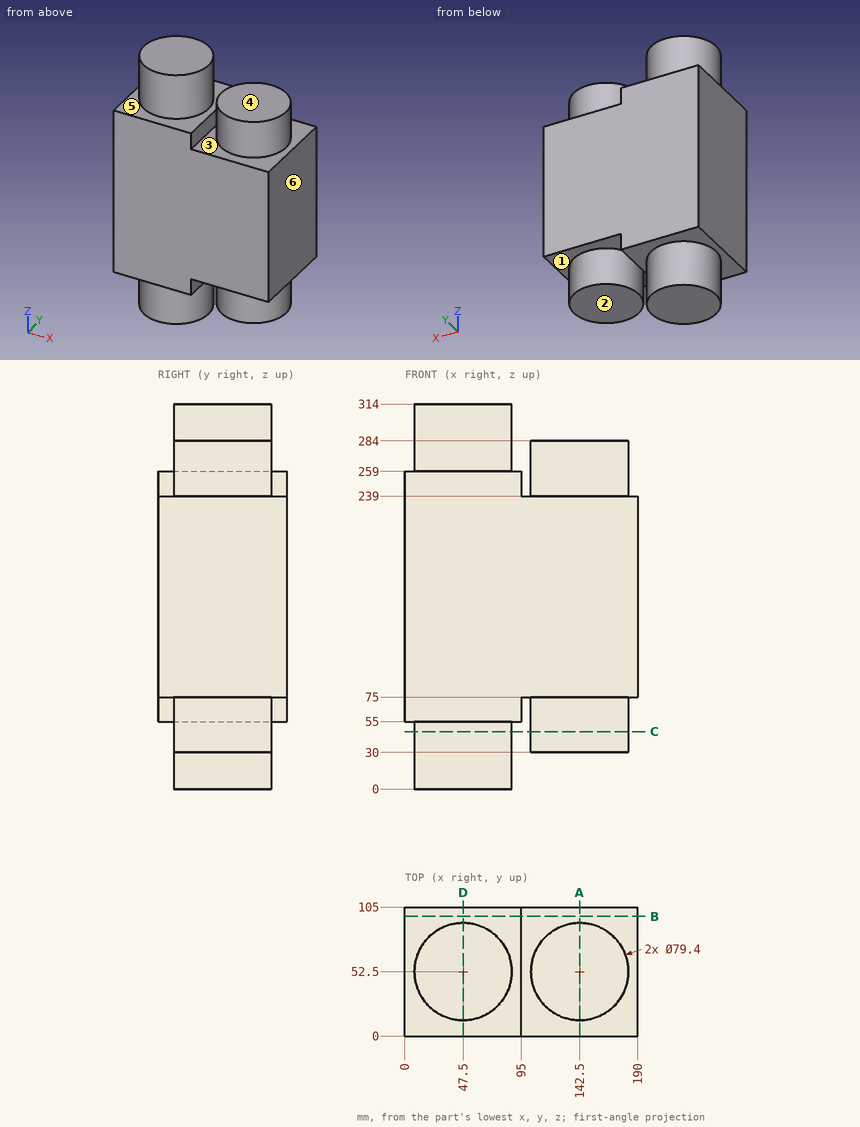
Source: three-view drawing plus pictorial views. Frame: mm from the lowest corner of the part. A direction names the side the tool comes from. Coordinates: 2 decimals unless noted, no trailing zeros. Order: outer loops, then holes, each group sorted by start corner. A loop starts at its lowest first (then second) coordinate and runs counter-clockwise, first axis right, second up. Notation, with made-up numbers: M 83.25,85 L 122.25,85 A27 cw 122.25,116 Z; hole C 56,15 d7. An arc over 180 degrees is marked long. Write each question's results on one line, items separated by ' | '. Start each with the question number.
1. Material intervals for L1, parallel to Z at x = 108, y = 78; L2, parallel to Z at x = 133, y = 40.5; L3, parallel to X at y = 56, z = 255, sorted ascending.
2. Section B-B, the plane y = 97.5. Return the cut outline in (x, z), then the cut area to 3 significant figures.
3. Section C-C, the plane z = 47. Return the cut outline in (x, y).
4. Section D-D, the plane x = 47.5. Return the cut outline in (y, z).
5. Draft query along X for the marked faces 4, 5 and 6. Return one class per face: +X half, -X half, draft (parallel to the pull), parting line (faces both ways), or undercut.
6. Section A-A, the plane x = 142.5. Return the cut outline in (y, z).
7. Pin query (flat end, axial travel): pin 1 (10 mm diameter, centred on y = 70.5, z = 248, fed in from +X); pin 2 (16 mm diameter, centred on y = 55.5, z = 63, fed in from +X); pin 3 (10 mm diameter, centred on x = 59, y = 25, fed in from -Z); pin 4 (24 mm diameter, centred on x = 132, y = 49, fed in from +Z). Return the tip coordinate at first contact, or that it passes through.
8. Reachability of the marked faces 1, 2 and 3 from +Z, -Z, +X, -X, +Y, -Y: full face, straight path, thin tool, end or side. Return the list, or none.
Solution:
1) L1: 75 to 239 | L2: 30 to 284 | L3: 0 to 95, 102.95 to 182.05
2) outline: M 0,55 L 95,55 L 95,75 L 190,75 L 190,239 L 95,239 L 95,259 L 0,259 Z | area: 35,000 mm²
3) outline: C 47.5,52.5 d79.4; C 142.5,52.5 d79.4
4) outline: M 0,55 L 12.8,55 L 12.8,0 L 92.2,0 L 92.2,55 L 105,55 L 105,259 L 92.2,259 L 92.2,314 L 12.8,314 L 12.8,259 L 0,259 Z
5) face 4: draft | face 5: undercut | face 6: +X half
6) outline: M 0,75 L 12.8,75 L 12.8,30 L 92.2,30 L 92.2,75 L 105,75 L 105,239 L 92.2,239 L 92.2,284 L 12.8,284 L 12.8,239 L 0,239 Z
7) pin 1: x = 180.01 | pin 2: x = 182.2 | pin 3: z = 0 | pin 4: z = 284
8) face 1: -Z | face 2: -Z, +X, +Y, -Y | face 3: +Z
